```python
from build123d import *

# Parameters (mm, degrees)
SKETCH1_R           = 4.7
BOSS_EXTRUDE1_DEPTH = 4
SKETCH2_R           = 3.5
BOSS_EXTRUDE2_DEPTH = 6.5
SKETCH3_R           = 2.75
BOSS_EXTRUDE3_DEPTH = 1
SKETCH4_R           = 3.5
BOSS_EXTRUDE4_DEPTH = 2.5
SKETCH5_R           = 2.5
CUT_EXTRUDE1_DEPTH  = 16.497741771


with BuildPart() as part:
    # Sketch1 → Boss-Extrude1 (new body)
    with BuildSketch(Plane(origin=(0, 0, 0), x_dir=(1, 0, 0), z_dir=(0, 1, 0))):
        with Locations(Location((0, 0, 0), (0, 0, 270))):
            Circle(SKETCH1_R)
    extrude(amount=BOSS_EXTRUDE1_DEPTH)

    # Sketch2 → Boss-Extrude2 (add)
    with BuildSketch(Plane(origin=(0, 4, 0), x_dir=(1, 0, 0), z_dir=(0, 1, 0))):
        with Locations(Location((0, 0, 0), (0, 0, 90))):
            Circle(SKETCH2_R)
    extrude(amount=BOSS_EXTRUDE2_DEPTH)

    # Sketch3 → Boss-Extrude3 (add)
    with BuildSketch(Plane(origin=(0, 10.5, 0), x_dir=(1, 0, 0), z_dir=(0, 1, 0))):
        with Locations(Location((0, 0, 0), (0, 0, 270))):
            Circle(SKETCH3_R)
    extrude(amount=BOSS_EXTRUDE3_DEPTH)

    # Sketch4 → Boss-Extrude4 (add)
    with BuildSketch(Plane(origin=(0, 11.5, 0), x_dir=(1, 0, 0), z_dir=(0, 1, 0))):
        with Locations(Location((0, 0, 0), (0, 0, 90))):
            Circle(SKETCH4_R)
    extrude(amount=BOSS_EXTRUDE4_DEPTH)

    # Sketch5 → Cut-Extrude1 (cut, through all)
    with BuildSketch(Plane(origin=(0, 14, 0), x_dir=(1, 0, 0), z_dir=(0, 1, 0))):
        with Locations(Location((0, 0, 0), (0, 0, 270))):
            Circle(SKETCH5_R)
    extrude(amount=-CUT_EXTRUDE1_DEPTH, mode=Mode.SUBTRACT)


solid = part.part
```
Source: CAD feature listing. Evaluate the final solid. Frame: model axes, mm. A direction names the side the tool comes from. Round coordinates to 2 decimals unless told otherwise and drop trailing zeros. Loops run counter-clockwise (first coordinate to the right, second up) from the corner with the lowest first, then second, coordinate; pieces in that order, holes last. Notation, with made-up numbers: M -19,11 L 21,11 A10 ccw 21,24 Z; hole C -35.75,-27.5 d5. An arc over 180 degrees is marked long. Use a Markdown table: item, result. Add a question column.
1. Section query B-B on z = 0. Return the cut outline in (x, y), then the cut area to 3 significant figures.
2. Reachability of faces 5 (the cylindrical face through (-2.44, 7.1, -0.54)), 6 (the flat face through (1, 11.5, 3)), 7 (the cylindrical face through (3.417, 7.204, 0.759)) from +Z, -Z, +X, -X, +Y, -Y: full face, straight path, thin tool, end or side. Return the list, or none.
3. Mould query, pull axis Y, two halves, no side actions, for faces 1 (the cylindrical face through (-2.685, 10.993, -0.596)), 2 (the cylindrical face through (3.417, 12.732, 0.759)), 3 (the flat face through (4, 4, 0)), 4 (the flat face through (1, 10.5, 3)). Classes: pulls with the +Y half, pulls with the -Y half, needs draft (parallel to the pull), parting line crosses it, or undercut.
4. Section query A-A on x = 0. Return the cut outline in (y, z), then the cut area to 3 significant figures.
5. Section query D-D on z = -3.25. Return the cut outline in (x, y), then the cut area to 3 significant figures.
6. Section query C-C on y = 11.25. Return the cut outline in (x, z).
7. Line query: line 1 (X direction, y = 11, z = 0); line 2 (X direction, y = 10.25, z = 0); line 3 (Y direction, x = 3, z = -1.75). Output: solid intervals per line, ascending.
8. Contact query for flat-ended pins moving along their axis: P1, Ø2, axis at x = 3.5, z = 1.5, coming from the +Y side; P2, Ø5, axis at y = 8.5, z = 2.5, coming from the +X side; P3, Ø3, axis at y = 7.5, z = -3, coming from the +X side; P4, Ø1.5, axis at y = 2, z = 1, coming from the -X side. Output: stop coordinate, or through.
Reported:
| question | item | result |
|---|---|---|
| 1 | outline | M -4.7,0 L -2.5,0 L -2.5,14 L -3.5,14 L -3.5,11.5 L -2.75,11.5 L -2.75,10.5 L -3.5,10.5 L -3.5,4 L -4.7,4 Z; M 2.5,0 L 4.7,0 L 4.7,4 L 3.5,4 L 3.5,10.5 L 2.75,10.5 L 2.75,11.5 L 3.5,11.5 L 3.5,14 L 2.5,14 Z |
| 1 | area | 36.1 mm² |
| 2 | face 5 | +Y, -Y |
| 2 | face 6 | none |
| 2 | face 7 | +Y |
| 3 | face 1 | undercut |
| 3 | face 2 | needs draft |
| 3 | face 3 | pulls with the +Y half |
| 3 | face 4 | undercut |
| 4 | outline | M 0,-4.7 L 4,-4.7 L 4,-3.5 L 10.5,-3.5 L 10.5,-2.75 L 11.5,-2.75 L 11.5,-3.5 L 14,-3.5 L 14,-2.5 L 0,-2.5 Z; M 0,2.5 L 14,2.5 L 14,3.5 L 11.5,3.5 L 11.5,2.75 L 10.5,2.75 L 10.5,3.5 L 4,3.5 L 4,4.7 L 0,4.7 Z |
| 4 | area | 36.1 mm² |
| 5 | outline | M -3.4,0 L 3.4,0 L 3.4,4 L 1.3,4 L 1.3,10.5 L -1.3,10.5 L -1.3,4 L -3.4,4 Z; M -1.3,11.5 L 1.3,11.5 L 1.3,14 L -1.3,14 Z |
| 5 | area | 50.5 mm² |
| 6 | outline | C 0,0 d5.5; hole C 0,0 d5 |
| 7 | line 1 | x = -2.75 to -2.5, 2.5 to 2.75 |
| 7 | line 2 | x = -3.5 to -2.5, 2.5 to 3.5 |
| 7 | line 3 | y = 0 to 10.5, 11.5 to 14 |
| 8 | P1 | stops at y = 14 |
| 8 | P2 | stops at x = 3.5 |
| 8 | P3 | stops at x = 3.16 |
| 8 | P4 | stops at x = -4.69 |
